Can you work these out from the model? Positions are in its coordinate system, mm. A direction names the side the tool comes from. Coordinates: 2 decimals unless noted, no trailing zeros. Order: outer loops, then holes, each group sorted by start corner. A loop starts at its lowest first (then second) coordinate and runs counter-clockwise, first axis right, second up. Notation, with made-up numbers: M -25,-15 L -19,-15 A24 ccw -19,-1 Z; hole C -32,78.5 d11. An arc over 180 degrees is marked long. Answer as a JSON object with one key per item and string values.
from build123d import *

# Parameters (mm, degrees)
F1_DEPTH = 76.2
F3_D     = 19.05
F4_R     = 9.525


with BuildPart() as f1:
    # F0 (on Top) → F1 (new body)
    with BuildSketch(Plane.XY):
        with BuildLine():
            Line((0, 67.9980737937), (0, 0))
            Line((0, 0), (31.75, 0))
            Line((31.75, 0), (31.75, 12.7))
            Line((31.75, 12.7), (12.7, 12.7))
            Line((12.7, 12.7), (12.7, 78.867))
            ThreePointArc((12.7, 78.867), (-19.558, 111.125), (12.7, 143.383))
            Line((12.7, 143.383), (12.7, 209.55))
            Line((12.7, 209.55), (31.75, 209.55))
            Line((31.75, 209.55), (31.75, 222.25))
            Line((31.75, 222.25), (0, 222.25))
            Line((0, 222.25), (0, 154.2519262063))
            ThreePointArc((0, 154.2519262063), (-32.258, 111.125), (0, 67.9980737937))
        make_face()
    extrude(amount=F1_DEPTH)

    # F3 (through all)
    with Locations(Plane(origin=(0, 0, 0), x_dir=(0, 1, 0), z_dir=(-1, 0, 0))):
        with Locations((187.0478298216, -38.1), (34.6478298216, -38.1)):
            Hole(F3_D / 2)

    # F4
    f4_edges = [f1.edges().sort_by_distance(p)[0] for p in [
        (0, 67.998074, 38.1),
        (0, 154.251926, 38.1),
        (0, 0, 38.1),
        (31.75, 6.35, 76.2),
        (31.75, 6.35, 0),
        (31.75, 215.9, 76.2),
        (31.75, 215.9, 0),
        (0, 222.25, 38.1),
    ]]
    fillet(f4_edges, radius=F4_R)


solid = f1.part
Item 1: If we mould it in two halves opening along Y, with no side actions, what happens to faces 1 (the flat face through (-19, 103, 76.2)), 2 (the flat face through (12.7, 176, 38)), 3 (the cylindrical face through (2.72, 219.39, 38.63))? For each: pulls with the +Y half, pulls with the -Y half, needs draft (parallel to the pull), parting line crosses it, or undercut.
Answers follow:
{"face 1": "needs draft", "face 2": "undercut", "face 3": "pulls with the +Y half"}
Item 2: I want a section at C-C, the plane z = 38.1. Write out the boundary of the cut face in (x, y) (3 decimals).
Answers follow:
{"outline": "M -5.64,70.078 A9.525 cw 0,61.381 L 0,44.173 L 12.7,44.173 L 12.7,78.867 A32.258 cw 12.7,143.383 L 12.7,177.523 L 0,177.523 L 0,160.869 A9.525 cw -5.64,152.172 A44.958 ccw Z; M 0,9.525 A9.525 ccw 9.525,0 L 31.75,0 L 31.75,12.7 L 12.7,12.7 L 12.7,25.123 L 0,25.123 Z; M 0,196.573 L 12.7,196.573 L 12.7,209.55 L 31.75,209.55 L 31.75,222.25 L 9.525,222.25 A9.525 ccw 0,212.725 Z"}
Item 3: Please list where these lines run through material, in increasing order: line 1 (Y direction, x = 6.25, z = 38.1); line 2 (Y direction, x = 17.5, z = 67); line 3 (Y direction, x = 4.5, z = 38.1).
Answers follow:
{"line 1": "y = 0.58 to 25.12, 44.17 to 79.52, 142.73 to 177.52, 196.57 to 221.67", "line 2": "y = 0 to 12.7, 209.55 to 222.25", "line 3": "y = 1.43 to 25.12, 44.17 to 79.93, 142.32 to 177.52, 196.57 to 220.82"}
Item 4: I want a section at B-B, the plane y = 36. Write out the boundary of the cut face in (x, z).
Answers follow:
{"outline": "M 0,0 L 12.7,0 L 12.7,28.67 L 0,28.67 Z; M 0,47.53 L 12.7,47.53 L 12.7,76.2 L 0,76.2 Z"}
Item 5: I want a section at A-A, the plane x = 2. Write out the boundary of the cut face in (y, z) (3 decimals).
Answers follow:
{"outline": "M 3.685,0 L 80.693,0 L 80.693,76.2 L 3.685,76.2 Z; M 141.557,0 L 218.565,0 L 218.565,76.2 L 141.557,76.2 Z; hole C 34.648,38.1 d19.05; hole C 187.048,38.1 d19.05"}
Item 6: Which directions (+Z, -Z, +X, -X, +Y, -Y) give clear straight access to the entire face, cutting with the end or side of a thin tool? Please do faces 4 (the flat face through (0, 42, 29)), 5 (the flat face through (0, 181, 46)), 6 (the flat face through (31.75, 6, 38)), 7 (the cylindrical face through (28.89, 215.99, 73.48)), 8 (the flat face through (12.7, 45, 38)).
Answers follow:
{"face 4": "+Z, -Z, -X, -Y", "face 5": "+Z, -Z, -X, +Y", "face 6": "+Z, -Z, +X, +Y, -Y", "face 7": "+Z, +X, +Y, -Y", "face 8": "+Z, -Z, +X"}
Item 7: I'm going to push flat-ended pins straight in: pin 1 (15.5 mm diameter, centred on y = 39, z = 29, fed in from -X); pin 2 (3 mm diameter, centred on y = 67.5, z = 65.5, fed in from +X); pin 3 (5 mm diameter, centred on x = -3.5, z = 11.5, fed in from +Y). Where does each tip first touch, or does it pass through?
Answers follow:
{"pin 1": "stops at x = 0", "pin 2": "stops at x = 12.7", "pin 3": "stops at y = 156.62"}
Item 8: I want a section at D-D, the plane x = 19.5. Write out the boundary of the cut face in (y, z), plus the area to 3 significant figures.
Answers follow:
{"outline": "M 0,0 L 12.7,0 L 12.7,76.2 L 0,76.2 Z; M 209.55,0 L 222.25,0 L 222.25,76.2 L 209.55,76.2 Z", "area": "1,940 mm^2"}
